Geometry: see drawing. Coordinates: mm, zero at the bounding-box minimum. A direction names the side the tool comes from. Give positions to 0.01 mm unless a question says otherwise; leave off trailing zeros. Loops run counter-clockwise (first coordinate to the right, second up) from the corner with the lowest first, then second, coordinate; pieces in that order, holes last. Notation, with made-up numbers: (80.25, 5.5) - (117.25, 5.5) arc R9 cw to (117.25, 19.5) - close; hole circle Ø10 at (0.5, 33). An arc over 180 degrees is marked (long way). Use CSV: the item, a comma, the result in double quotes. Start each with the question number.
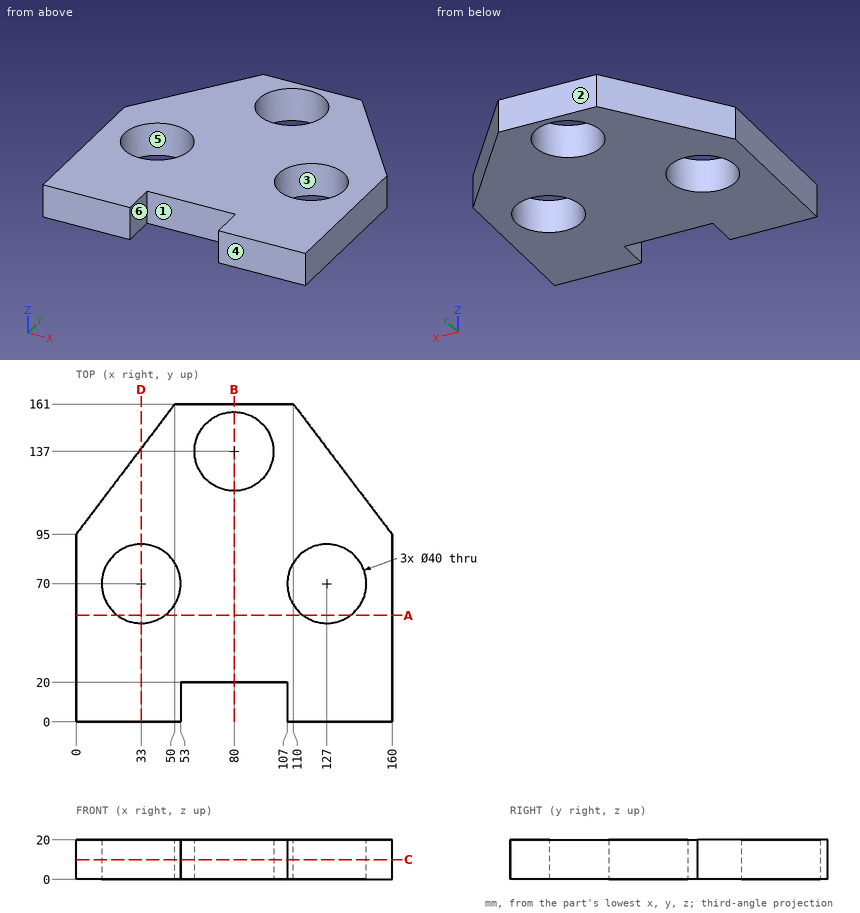
Item 1: Pin query (flat end, axial travel): pin 1 Ø24 at (x, y) = (80, 137) entering from -Z; pin 2 Ø4 at (x, z) = (28.5, 8.5) entering from +Y; pin 3 Ø12 at (x, z) = (72.5, 17) entering from -Y. Return the tip coordinate at first contact, or that it passes through.
Item 2: Section B-B (x = 80). Output: boundary loops of the cut face in (y, z), plus the area to 3 significant figures.
Item 3: Reachability of the marked faces 1 and 2 from +Z, -Z, +X, -X, +Y, -Y: full face, straight path, thin tool, end or side. Return the list, or none.
Item 4: Section D-D (x = 33). Output: boundary loops of the cut face in (y, z).
Item 5: Ray query, probe 1 along Y at (x, z) = (80, 2); probe 2 along X at (y, z) = (14, 14.5); probe 3 along X at (y, z) = (52.5, 13.25). Return the intervals inside material, ascending.
Item 6: Section C-C (z = 10). Output: boundary loops of the cut face in (x, y), plus the area to 3 significant figures.
Item 7: Section A-A (y = 54). Output: boundary loops of the cut face in (x, z).
Item 8: Mould query, pull axis Y, two halves, no side actions, for the marked faces 3, 4, 5 and 6. Classes: pulls with the +Y half, pulls with the -Y half, needs draft (parallel to the pull), parting line crosses it, or undercut.
Outcome:
1,pin 1,"passes through"
1,pin 2,"stops at y = 135.26"
1,pin 3,"stops at y = 20"
2,outline,"(20, 0) - (117, 0) - (117, 20) - (20, 20) - close; (157, 0) - (161, 0) - (161, 20) - (157, 20) - close"
2,area,"2,020 mm2"
3,face 1,"+Z, -Z, -Y"
3,face 2,"+Z, -Z, +X, -X, +Y"
4,outline,"(0, 0) - (50, 0) - (50, 20) - (0, 20) - close; (90, 0) - (138.56, 0) - (138.56, 20) - (90, 20) - close"
5,probe 1,"y = 20 to 117, 157 to 161"
5,probe 2,"x = 0 to 53, 107 to 160"
5,probe 3,"x = 0 to 23.32, 42.68 to 117.32, 136.68 to 160"
6,outline,"(0, 0) - (53, 0) - (53, 20) - (107, 20) - (107, 0) - (160, 0) - (160, 95) - (110, 161) - (50, 161) - (0, 95) - close; hole circle Ø40 at (33, 70); hole circle Ø40 at (80, 137); hole circle Ø40 at (127, 70)"
6,area,"17,600 mm2"
7,outline,"(0, 0) - (21, 0) - (21, 20) - (0, 20) - close; (45, 0) - (115, 0) - (115, 20) - (45, 20) - close; (139, 0) - (160, 0) - (160, 20) - (139, 20) - close"
8,face 3,"undercut"
8,face 4,"pulls with the -Y half"
8,face 5,"undercut"
8,face 6,"needs draft"
